Can you work these out from the model? Positions are in its coordinate system, mm. Coordinates: 2 decimals unless noted, no trailing zeros. Order: outer loops, then holes, each group sorted by start corner. A loop starts at its lowest first (then second) coordinate and runs counter-clockwise, first axis right, second up. Notation, with made-up numbers: (-13.5, 23) - (-7.5, 23) arc R9 cw to (-7.5, 33) - close; hole circle Ø6 at (87, -27.5). An arc over 180 degrees is marked (long way). Use a Markdown table: item, result. Add a question column.
(1) I want a section at C-C (y = -73). List the corners of the cut face in (x, z) for me.
(2) If I drill on L1, parallel to Z at x = 1, y = -18; L2, parallel to Y at x = 6, z = 136; L3, parallel to Y at x = 11, z = 178.5, over which ranges is the centre line in solid material (lowest first)? Write a range as [from, to].
(3) For pin 1 Ø4 at (x, z) = (5, 19) entering from +Y; pin 2 Ø2 at (x, y) = (1.5, -86) entering from +Z; pin 3 Ø4 at (x, z) = (9, 250.5) entering from +Y, each with a flat end and sliding along its axis, tell me the tip position at first contact or that it passes through.
(4) I want a section at D-D (z = 305.5). List the corners of the cut face in (x, y) for me.
(5) I want a section at A-A (y = -9). List the corners of the cut face in (x, z) for me, and give its area (3 significant figures).
(6) I want a section at B-B (x = 9.25). State how many separate pieces and enclosed holes the cut face has, and give its area (3 significant figures).
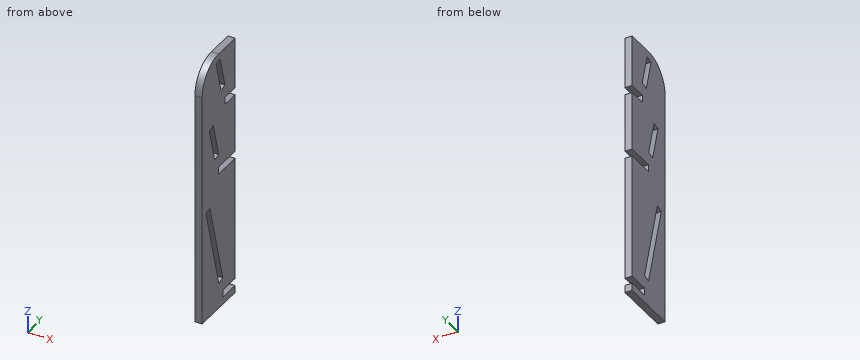
```python
from build123d import *

# Parameters (mm, degrees)
F1_DEPTH = 12.7


with BuildPart() as f1:
    # F0 (on Right) → F1 (new body)
    with BuildSketch(Plane.YZ):
        with BuildLine():
            Line((-101.6, 0), (0, 0))
            Line((0, 0), (0, 12.7))
            Line((0, 12.7), (-38.1, 12.7))
            Line((-38.1, 12.7), (-38.1, 25.4))
            Line((-38.1, 25.4), (0, 25.4))
            Line((0, 25.4), (0, 241.3))
            Line((0, 241.3), (-50.8, 241.3))
            Line((-50.8, 241.3), (-50.8, 254))
            Line((-50.8, 254), (0, 254))
            Line((0, 254), (0, 355.6))
            Line((0, 355.6), (-31.75, 355.6))
            Line((-31.75, 355.6), (-31.75, 368.3))
            Line((-31.75, 368.3), (0, 368.3))
            Line((0, 368.3), (0, 457.2))
            Line((0, 457.2), (-50.8, 457.2))
            ThreePointArc((-50.8, 457.2), (-86.721024, 442.321024), (-101.6, 406.4))
            Line((-101.6, 406.4), (-101.6, 0))
        make_face()
        Polygon((-77.544022, 194.944098), (-38.1, 47.737002), (-50.367258, 44.45), (-89.81128, 191.657096), align=None, mode=Mode.SUBTRACT)
        Polygon((-63.067258, 273.05), (-79.502267, 334.38629), (-67.235009, 337.673292), (-50.8, 276.337002), align=None, mode=Mode.SUBTRACT)
        Polygon((-43.65244, 387.35), (-58.443948, 442.552661), (-46.17669, 445.839663), (-31.385182, 390.637002), align=None, mode=Mode.SUBTRACT)
    extrude(amount=F1_DEPTH)


solid = f1.part
```
Answers follow:
| question | item | result |
|---|---|---|
| 1 | outline | (0, 0) - (12.7, 0) - (12.7, 128.92) - (0, 128.92) - close; (0, 177.99) - (12.7, 177.99) - (12.7, 310.12) - (0, 310.12) - close; (0, 336.13) - (12.7, 336.13) - (12.7, 452.09) - (0, 452.09) - close |
| 2 | L1 | z = [0, 12.7], [25.4, 241.3], [254, 355.6], [368.3, 457.2] |
| 2 | L2 | y = [-101.6, -74.9], [-61.75, 0] |
| 2 | L3 | y = [-101.6, -86.29], [-73.14, 0] |
| 3 | pin 1 | stops at y = -38.1 |
| 3 | pin 2 | stops at z = 443.96 |
| 3 | pin 3 | stops at y = -50.8 |
| 4 | outline | (0, -101.6) - (12.7, -101.6) - (12.7, -71.76) - (0, -71.76) - close; (0, -58.61) - (12.7, -58.61) - (12.7, 0) - (0, 0) - close |
| 5 | outline | (0, 0) - (12.7, 0) - (12.7, 12.7) - (0, 12.7) - close; (0, 25.4) - (12.7, 25.4) - (12.7, 241.3) - (0, 241.3) - close; (0, 254) - (12.7, 254) - (12.7, 355.6) - (0, 355.6) - close; (0, 368.3) - (12.7, 368.3) - (12.7, 457.2) - (0, 457.2) - close |
| 5 | area | 5,320 mm² |
| 6 | separate pieces | 1 |
| 6 | enclosed holes | 3 |
| 6 | area | 40,900 mm² |
